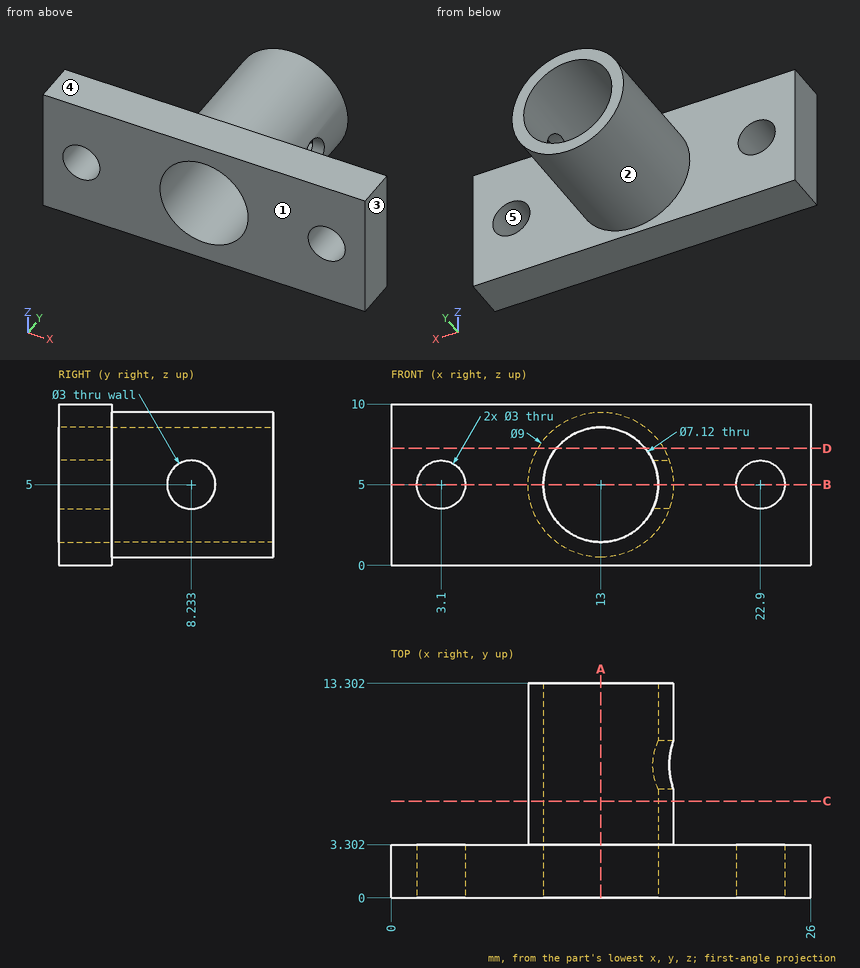
Check sheet for the drawn part. Datum: minimum x, y, z corner. Units: mm. A direction names the side the tool comes from. Coordinates: 2 decimals unless noted, no trailing zeros. Loops run counter-clockwise (first coordinate to the right, second up) from the corner with the lowest first, then second, coordinate; pieces in that order, holes last. Notation, with made-up numbers: (74, 87.25) -> (130, 87.25) arc R6 ccw to (130, 95.25) -> close; hole circle Ø6 at (70, -4). An arc over 180 degrees is marked (long way). Answer in a Markdown table with one row per item.
1) Section check B-B (z = 5). Record the cut outline in (x, y).
The answers:
| item | result |
|---|---|
| outline | (0, 0) -> (1.6, 0) -> (1.6, 3.3) -> (0, 3.3) -> close; (4.6, 0) -> (9.44, 0) -> (9.44, 13.3) -> (8.5, 13.3) -> (8.5, 3.3) -> (4.6, 3.3) -> close; (16.56, 0) -> (21.4, 0) -> (21.4, 3.3) -> (17.5, 3.3) -> (17.5, 6.73) -> (16.56, 6.73) -> close; (16.56, 9.73) -> (17.5, 9.73) -> (17.5, 13.3) -> (16.56, 13.3) -> close; (24.4, 0) -> (26, 0) -> (26, 3.3) -> (24.4, 3.3) -> close |
2) Section check A-A (x = 13). Record the cut outline in (y, z), and give its area (3 significant figures).
The answers:
| item | result |
|---|---|
| outline | (0, 0) -> (3.3, 0) -> (3.3, 0.5) -> (13.3, 0.5) -> (13.3, 1.44) -> (0, 1.44) -> close; (0, 8.56) -> (13.3, 8.56) -> (13.3, 9.5) -> (3.3, 9.5) -> (3.3, 10) -> (0, 10) -> close |
| area | 28.3 mm2 |
3) Access from +Z, -Z, +X, -X, +Y, -Y to the whole of each face (thin tool, end or side, straight path). Record for the marked faces 1 and 2.
The answers:
| item | result |
|---|---|
| face 1 | +Z, -Z, +X, -X, -Y |
| face 2 | +Y |
4) Depth check by flat-ended pin: P1, Ø2.5, axis at x = 22.9, z = 5, coming from the +Y side; P2, Ø5, axis at y = 8.23, z = 5, coming from the -X side. Enter the tip coordinate at first touch or a pass-through.
The answers:
| item | result |
|---|---|
| P1 | passes through |
| P2 | stops at x = 8.5 |
5) Section check C-C (y = 6). Record the cut outline in (x, z), and give its area (3 significant figures).
The answers:
| item | result |
|---|---|
| outline | circle Ø9 at (13, 5); hole circle Ø7.12 at (13, 5) |
| area | 23.8 mm2 |
6) Scan lines: line 1 along X through (y, z) = (1.75, 5); line 2 along X through (y, z) = (3, 6.25) (1 decimal); line 3 along Y through (x, z) = (16.6, 5). Record each from-to range of solid material in increasing order. Write a range as from..to.
The answers:
| item | result |
|---|---|
| line 1 | x = 0..1.6, 4.6..9.44, 16.56..21.4, 24.4..26 |
| line 2 | x = 0..2.3, 3.9..9.7, 16.3..22.1, 23.7..26 |
| line 3 | y = 0..6.73, 9.73..13.3 |
7) Section check D-D (z = 7.25). Record the cut outline in (x, y).
The answers:
| item | result |
|---|---|
| outline | (0, 0) -> (10.24, 0) -> (10.24, 13.3) -> (9.1, 13.3) -> (9.1, 3.3) -> (0, 3.3) -> close; (15.76, 0) -> (26, 0) -> (26, 3.3) -> (16.9, 3.3) -> (16.9, 13.3) -> (15.76, 13.3) -> close |
8) Draft check along X on the marked faces 3, 4 and 5. Enter one of: released by +X, released by -X, zero draft, split by the parting line, or undercut.
The answers:
| item | result |
|---|---|
| face 3 | released by +X |
| face 4 | zero draft |
| face 5 | undercut |
